```python
from build123d import *

# Parameters (mm, degrees)
SKETCH1_W           = 114
SKETCH1_H           = 114
SKETCH1_R           = 1.5
BOSS_EXTRUDE1_DEPTH = 1.5
SKETCH2_W           = 10
SKETCH2_H           = 5
BOSS_EXTRUDE2_DEPTH = 72
SKETCH3_W           = 27
SKETCH3_H           = 10
SKETCH3_R           = 1.5
BOSS_EXTRUDE3_DEPTH = 5


with BuildPart() as part:
    # Sketch1 → Boss-Extrude1 (new body)
    with BuildSketch(Plane(origin=(0, 0, 0), x_dir=(1, 0, 0), z_dir=(0, 1, 0))):
        Rectangle(SKETCH1_W, SKETCH1_H)
        with Locations((29.5, 5)):
            Circle(SKETCH1_R, mode=Mode.SUBTRACT)
        with Locations((49.5, 5)):
            Circle(SKETCH1_R, mode=Mode.SUBTRACT)
        with Locations((-29.5, -46)):
            Circle(SKETCH1_R, mode=Mode.SUBTRACT)
        with Locations((-49.5, -46)):
            Circle(SKETCH1_R, mode=Mode.SUBTRACT)
    extrude(amount=BOSS_EXTRUDE1_DEPTH)

    # Sketch2 → Boss-Extrude2 (add)
    with BuildSketch(Plane(origin=(0, 1.5, 0), x_dir=(1, 0, 0), z_dir=(0, 1, 0))):
        with Locations((-39.5, -46)):
            Rectangle(SKETCH2_W, SKETCH2_H)
        with Locations((39.5, 5)):
            Rectangle(SKETCH2_W, SKETCH2_H)
    extrude(amount=-BOSS_EXTRUDE2_DEPTH)

    # Sketch3 → Boss-Extrude3 (add)
    with BuildSketch(Plane(origin=(0, -70.5, 0), x_dir=(-1, 0, 0), z_dir=(0, -1, 0))):
        with Locations((39.5, -46)):
            Rectangle(SKETCH3_W, SKETCH3_H)
        with Locations((49.5, -46)):
            Circle(SKETCH3_R, mode=Mode.SUBTRACT)
        with Locations((29.5, -46)):
            Circle(SKETCH3_R, mode=Mode.SUBTRACT)
        with Locations((-39.5, 5)):
            Rectangle(SKETCH3_W, SKETCH3_H)
        with Locations((-29.5, 5)):
            Circle(SKETCH3_R, mode=Mode.SUBTRACT)
        with Locations((-49.5, 5)):
            Circle(SKETCH3_R, mode=Mode.SUBTRACT)
    extrude(amount=BOSS_EXTRUDE3_DEPTH)


solid = part.part
```
For this review, take the finished solid that the model builds, in its own axes (mm). A direction names the side the tool comes from. Give positions to 0.01 mm unless a question says otherwise; leave off trailing zeros. Write each loop counter-clockwise with the first axis right and the second up, starting at its lowest first coordinate (ties: lowest second). Pieces come first, ordered by that corner, then holes. Notation, with made-up numbers: M 77,77.25 L 108,77.25 A28 cw 108,100.25 Z; hole C -17.75,38.5 d11. An arc over 180 degrees is marked long. Answer as CSV lines item,"result".
1. Consider section B-B, the plane z = 46. Write out the cut boundary in (x, y).
Findings:
outline,"M -57,0 L -51,0 L -51,1.5 L -57,1.5 Z; M -53,-75.5 L -51,-75.5 L -51,-70.5 L -53,-70.5 Z; M -48,-75.5 L -31,-75.5 L -31,-70.5 L -34.5,-70.5 L -34.5,0 L -31,0 L -31,1.5 L -48,1.5 L -48,0 L -44.5,0 L -44.5,-70.5 L -48,-70.5 Z; M -28,-75.5 L -26,-75.5 L -26,-70.5 L -28,-70.5 Z; M -28,0 L 57,0 L 57,1.5 L -28,1.5 Z"
2. Consider section D-D, the plane z = -24. Write out the cut boundary in (x, y), then the cut area to 3 significant figures.
Findings:
outline,"M -57,0 L 57,0 L 57,1.5 L -57,1.5 Z"
area,"171 mm2"
3. For faces 4 (the flat face through (-53, -73, 46)), 5 (the flat face through (39, -35, -7.5)), 6 (the flat face through (-40, -35, 48.5)), 7 (the flat face through (34.5, -35, -5)), 8 (the flat face through (-34.5, -35, 46)), list the 3-axis set-ups (+Z, -Z, +X, -X, +Y, -Y) from which the entire face can be reached by the end or side of a thin tool; tool diameter is ignored.
Findings:
face 4,"+Z, -Z, -X, -Y"
face 5,"-Z, +X, -X"
face 6,"+Z, +X, -X"
face 7,"+Z, -Z, -X"
face 8,"+Z, -Z, +X"
4. Wall thickness on line 1 (X direction, y = 1.2, z = -5); line 2 (X direction, y = -72.2, z = -5); line 3 (Z direction, x = -49.5, y = 0.75): over which ranges is each line inside the solid? List them lowest first.
Findings:
line 1,"x = -57 to 28, 31 to 48, 51 to 57"
line 2,"x = 26 to 28, 31 to 48, 51 to 53"
line 3,"z = -57 to 44.5, 47.5 to 57"
5. Consider section C-C, the plane y = -58.5. Write out the cut boundary in (x, z).
Findings:
outline,"M -44.5,43.5 L -34.5,43.5 L -34.5,48.5 L -44.5,48.5 Z; M 34.5,-7.5 L 44.5,-7.5 L 44.5,-2.5 L 34.5,-2.5 Z"
6. Consider section A-A, the plane x = 49.5. Write out the cut boundary in (y, z).
Findings:
outline,"M -75.5,-10 L -70.5,-10 L -70.5,-6.5 L -75.5,-6.5 Z; M -75.5,-3.5 L -70.5,-3.5 L -70.5,0 L -75.5,0 Z; M 0,-57 L 1.5,-57 L 1.5,-6.5 L 0,-6.5 Z; M 0,-3.5 L 1.5,-3.5 L 1.5,57 L 0,57 Z"
7. For pin 1 (6 mm diameter, centred on x = 44, y = -9, fed in from -Z); pin 2 (4 mm diameter, centred on x = -41.5, y = -73.5, fed in from -Z); pin 3 (5.5 mm diameter, centred on x = 43, y = -72, fed in from +Z); pin 4 (3.5 mm diameter, centred on x = 49.5, z = -5, fed in from +Y), all flat-tipped, find the tip position at first contact; note any pin that passes through.
Findings:
pin 1,"stops at z = -7.5"
pin 2,"stops at z = 41"
pin 3,"stops at z = 0"
pin 4,"stops at y = 1.5"
8. Draft analysis for pull direction Y (two halves, no side actions). For faces 1 (the flat face through (-40, -35, 43.5)), 2 (the flat face through (-1, 1.5, -1)), 3 (the flat face through (26, -73, -5)), state which applies: +Y half, -Y half, draft (parallel to the pull), parting line (faces both ways), or undercut.
Findings:
face 1,"undercut"
face 2,"+Y half"
face 3,"draft"
